Input: part model. Units: mm. Frame: model coordinates. Face numbers are marked on the shaded views. Coordinates: 2 decimals unless noted, no trailing zeros. Order: outer loops, then holes, each group sorted by start corner. A loop starts at its lowest first (then second) coordinate and runs counter-clockwise, first axis right, second up. Notation, with made-up numbers: (4, -33) -> (42, -33) arc R25 ccw to (42, -4) -> close; hole circle Ø3 at (-26, -16.75). An arc over 180 degrees is marked (long way). Write each question's results on one line, items separated by ' | '.
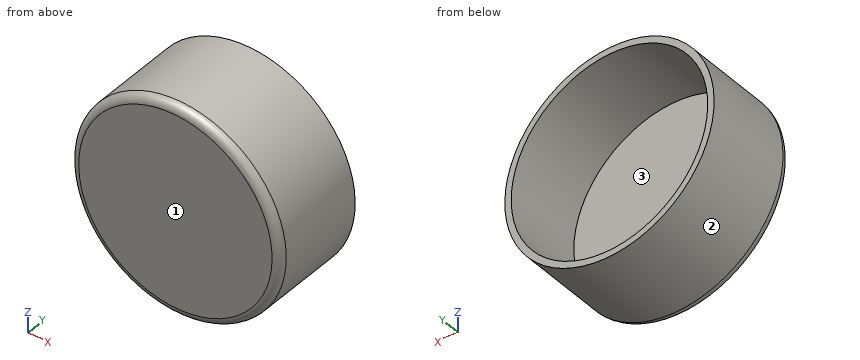
```python
from build123d import *

# Parameters (mm, degrees)
SKETCH1_R           = 13.15
BOSS_EXTRUDE1_DEPTH = 2
SKETCH2_R           = 13.15
SKETCH2_R_2         = 12.35
BOSS_EXTRUDE2_DEPTH = 10
FILLET1_R           = 1


with BuildPart() as part:
    # Sketch1 → Boss-Extrude1 (new body)
    with BuildSketch(Plane(origin=(0, 0, 0), x_dir=(1, 0, 0), z_dir=(0, 1, 0))):
        with Locations(Location((0, 0, 0), (0, 0, 270))):
            Circle(SKETCH1_R)
    extrude(amount=BOSS_EXTRUDE1_DEPTH)

    # Sketch2 → Boss-Extrude2 (add)
    with BuildSketch(Plane(origin=(0, 2, 0), x_dir=(1, 0, 0), z_dir=(0, 1, 0))):
        with Locations(Location((0, 0, 0), (0, 0, 270))):
            Circle(SKETCH2_R)
        with Locations(Location((0, 0, 0), (0, 0, 270))):
            Circle(SKETCH2_R_2, mode=Mode.SUBTRACT)
    extrude(amount=BOSS_EXTRUDE2_DEPTH)

    # Fillet1
    fillet1_edges = [part.edges().sort_by_distance(p)[0] for p in [
        (0, 0, -13.15),
    ]]
    fillet(fillet1_edges, radius=FILLET1_R)


solid = part.part
```
(1) Pin query (flat end, axial travel): P1, Ø6, axis at x = 6.5, z = 4, coming from the +Y side; P2, Ø4, axis at y = 9.5, z = -4, coming from the -X side; P3, Ø5, axis at x = -8, y = 6, coming from the -Z side. Return the tip coordinate at first contact, or that it passes through.
Return value:
P1: y = 2 | P2: x = -13 | P3: z = -11.94
(2) Line query: line 1 along X through (y, z) = (8.75, 0); line 2 along Y through (x, z) = (-9.5, 6); line 3 along X through (y, z) = (10.75, -3.5). Output: solid intervals per line, ascending. Write a range as from..to.
Return value:
line 1: -13.15..-12.35, 12.35..13.15 | line 2: 0..2 | line 3: -12.68..-11.84, 11.84..12.68
(3) Mould query, pull axis Z, two halves, no side actions, for the marked faces 1, 2 and 3. Classes: +Z half, -Z half, draft (parallel to the pull), parting line (faces both ways), or undercut.
Return value:
face 1: draft | face 2: parting line | face 3: undercut
(4) Cut plane B-B, the plane x = 0. Return loops of the section in (y, z).
Return value:
outline: (0, -12.15) arc R1 ccw to (1, -13.15) -> (12, -13.15) -> (12, -12.35) -> (2, -12.35) -> (2, 12.35) -> (12, 12.35) -> (12, 13.15) -> (1, 13.15) arc R1 ccw to (0, 12.15) -> close
(5) Cut plane C-C, the plane y = 10. Return loops of the section in (x, z).
Return value:
outline: circle Ø26.3 at (0, 0); hole circle Ø24.7 at (0, 0)
(6) Cut plane A-A, the plane z = 0. Return loops of the section in (x, y).
Return value:
outline: (-13.15, 1) arc R1 ccw to (-12.15, 0) -> (12.15, 0) arc R1 ccw to (13.15, 1) -> (13.15, 12) -> (12.35, 12) -> (12.35, 2) -> (-12.35, 2) -> (-12.35, 12) -> (-13.15, 12) -> close
